Verification items for the finished model (mm, model axes). Face numbers are marked on the shaded views. A direction names the side the tool comes from. Coordinates: 2 decimals unless noted, no trailing zeros. Order: outer loops, then holes, each group sorted by start corner. A loop starts at its lowest first (then second) coordinate and runs counter-clockwise, first axis right, second up. Notation, with made-up numbers: M 39,32.25 L 57,32.25 A24 cw 57,44.25 Z; hole C -1.5,-1.75 d9. An arc over 180 degrees is marked long. Answer as a JSON object with one key per item and string values. Group by question number.
(1) Cross-section at C-C (z = 10.5). Enter the section's corners in (x, y), plus the area to 3 significant figures.
(2) Material ranges on line 1 (Y direction, x = 32, z = 0.85); line 2 (Y direction, x = 12, z = 8.5); line 3 (X direction, y = 1.5, z = 3.5), recorded low to high.
(3) Access from +Z, -Z, +X, -X, +Y, -Y to the whole of each face (thin tool, end or side, straight path). Record for the marked faces 4, 5 and 6.
(4) Mould release check, pull along Y, two halves, no side actions. Record for the marked faces 1, 2 and 3: released by +Y, released by -Y, zero draft, split by the parting line, or undercut.
(5) Cross-section at B-B (x = 32). Enter the section's corners in (y, z), plus the area to 3 significant figures.
(6) Cross-section at D-D (y = 20.5). Enter the section's corners in (x, z).
(7) Gauge pin test, flat ends, axial feed: pin 1 Ø2.5 at (x, y) = (32, 20.5) entering from +Z; pin 2 Ø3.5 at (x, z) = (-31.5, 6.5) entering from -Y; pin 3 Ø6 at (x, y) = (9.5, -4.5) entering from +Z; pin 4 Ø1.8 at (x, z) = (33, 8.5) entering from -Y. Record the tip position at first contact, or that the pin passes through.
(8) Cross-section at A-A (z = 3.35). Enter the section's corners in (x, y), plus the area to 3 significant figures.
from build123d import *

# Parameters (mm, degrees)
ESBO_O1_W                = 70
ESBO_O1_H                = 47.2
ESBO_O1_R                = 1.6
RESSALTO_EXTRUS_O1_DEPTH = 1.6
ESBO_O2_W                = 49.366448858
ESBO_O2_H                = 6.785766069
ESBO_O2_W_2              = 54.120377738
ESBO_O2_H_2              = 7.496391297
ESBO_O2_W_3              = 5.916216247
ESBO_O2_H_3              = 28.306864236
ESBO_O2_W_4              = 7.279806524
ESBO_O2_H_4              = 17.669935009
RESSALTO_EXTRUS_O2_DEPTH = 10
RESSALTO_EXTRUS_O3_DEPTH = 7


with BuildPart() as part:
    # Esboço1 → Ressalto-extrusão1 (new body)
    with BuildSketch(Plane.XY):
        Rectangle(ESBO_O1_W, ESBO_O1_H)
        with Locations((-32, 20.5)):
            Circle(ESBO_O1_R, mode=Mode.SUBTRACT)
        with Locations((32, 20.5)):
            Circle(ESBO_O1_R, mode=Mode.SUBTRACT)
        with Locations((32, -20.5)):
            Circle(ESBO_O1_R, mode=Mode.SUBTRACT)
        with Locations((-32, -20.5)):
            Circle(ESBO_O1_R, mode=Mode.SUBTRACT)
    extrude(amount=RESSALTO_EXTRUS_O1_DEPTH)

    # Esboço2 → Ressalto-extrusão2 (add)
    with BuildSketch(Plane.XY.offset(1.6)):
        with Locations((3.036969047, -20.207116965)):
            Rectangle(ESBO_O2_W, ESBO_O2_H)
        with Locations((0, 19.851804352)):
            Rectangle(ESBO_O2_W_2, ESBO_O2_H_2)
        with Locations((32.041891877, 0)):
            Rectangle(ESBO_O2_W_3, ESBO_O2_H_3)
        with Locations((-31.360096738, 5.213703653)):
            Rectangle(ESBO_O2_W_4, ESBO_O2_H_4)
    extrude(amount=RESSALTO_EXTRUS_O2_DEPTH)

    # Esboço3 → Ressalto-extrusão3 (add)
    with BuildSketch(Plane.ZY.offset(35)):
        with BuildLine():
            Line((5.1, -9.35), (5.1, -14.85))
            ThreePointArc((5.1, -14.85), (3.35, -16.6), (1.6, -14.85))
            Line((1.6, -14.85), (1.6, -9.35))
            ThreePointArc((1.6, -9.35), (3.35, -7.6), (5.1, -9.35))
        make_face()
    extrude(amount=-RESSALTO_EXTRUS_O3_DEPTH)


solid = part.part
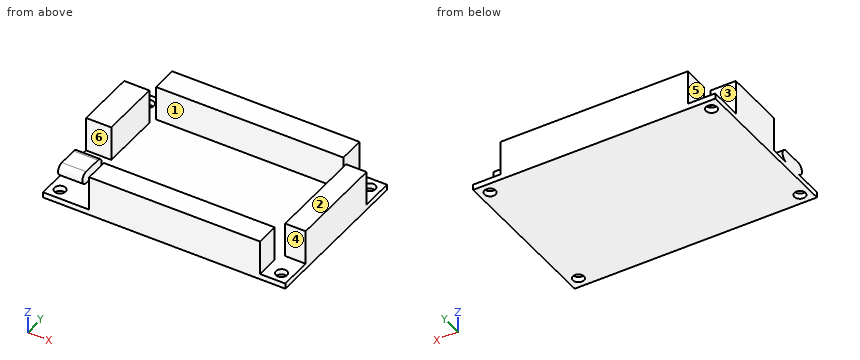
Taken from the geometry:
{
 "1": {"outline": "M -35,-3.62 L -27.72,-3.62 L -27.72,14.05 L -35,14.05 Z; M -27.06,16.1 L 27.06,16.1 L 27.06,23.6 L -27.06,23.6 Z; M -21.65,-23.6 L 27.72,-23.6 L 27.72,-16.81 L -21.65,-16.81 Z; M 29.08,-14.15 L 35,-14.15 L 35,14.15 L 29.08,14.15 Z", "area": "1,040 mm²"},
 "2": {"line 1": "y = -23.6 to -22.1, -18.9 to 18.9, 22.1 to 23.6", "line 2": "y = -23.6 to -16.81, 16.1 to 23.6", "line 3": "x = -35 to -27.72, 29.08 to 35"},
 "3": {"face 4": "+Z, +X, -Y", "face 5": "+Z, -X, +Y, -Y", "face 6": "+Z, -X"},
 "4": {"face 1": "undercut", "face 2": "zero draft", "face 3": "released by +Y"},
 "5": {"outline": "M -23.6,0 L -22.1,0 L -22.1,1.6 L -23.6,1.6 Z; M -18.9,0 L 18.9,0 L 18.9,1.6 L 14.15,1.6 L 14.15,11.6 L -14.15,11.6 L -14.15,1.6 L -18.9,1.6 Z; M 22.1,0 L 23.6,0 L 23.6,1.6 L 22.1,1.6 Z", "area": "348 mm²"},
 "6": {"outline": "M -35,0 L -33.6,0 L -33.6,1.6 L -35,1.6 Z; M -30.4,0 L 30.4,0 L 30.4,1.6 L 27.06,1.6 L 27.06,11.6 L -27.06,11.6 L -27.06,1.6 L -30.4,1.6 Z; M 33.6,0 L 35,0 L 35,1.6 L 33.6,1.6 Z"},
 "7": {"pin 1": "passes through", "pin 2": "stops at y = -15.9", "pin 3": "stops at z = 1.6", "pin 4": "stops at y = -14.15"},
 "8": {"outline": "M -35,-16.6 L -28,-16.6 L -28,-7.6 L -35,-7.6 Z; M -35,-3.62 L -27.72,-3.62 L -27.72,14.05 L -35,14.05 Z; M -27.06,16.1 L 27.06,16.1 L 27.06,23.6 L -27.06,23.6 Z; M -21.65,-23.6 L 27.72,-23.6 L 27.72,-16.81 L -21.65,-16.81 Z; M 29.08,-14.15 L 35,-14.15 L 35,14.15 L 29.08,14.15 Z", "area": "1,100 mm²"}
}
